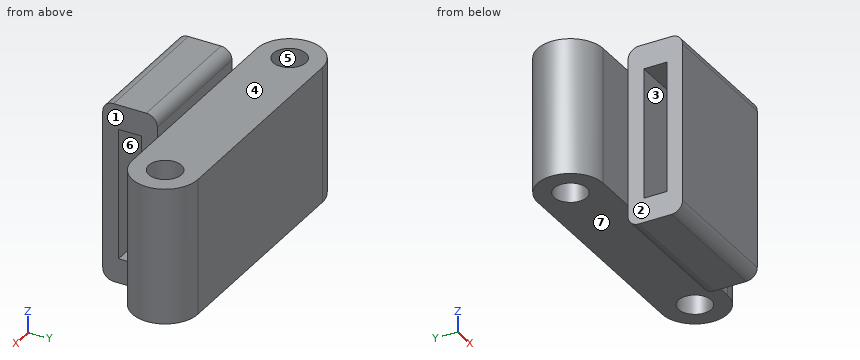
```python
from build123d import *

# Parameters (mm, degrees)
F0_W     = 12
F0_H     = 16.5
F1_DEPTH = 5
F2_R     = 1.5
F3_DEPTH = 6.25
F4_W     = 2.1
F4_H     = 12
F5_DEPTH = 12
F6_R     = 1


with BuildPart() as f1:
    # F0 (on Front) → F1 (new body)
    with BuildSketch(Plane.XZ):
        Rectangle(F0_W, F0_H)
    extrude(amount=F1_DEPTH)

    # F2 (on Top) → F3 (join, symmetric)
    with BuildSketch(Plane.XY):
        with BuildLine():
            Line((-10, 0), (10, 0))
            ThreePointArc((10, 0), (13, 3), (10, 6))
            Line((10, 6), (-10, 6))
            ThreePointArc((-10, 6), (-13, 3), (-10, 0))
        make_face()
        with Locations((-10, 3)):
            Circle(F2_R, mode=Mode.SUBTRACT)
        with Locations((10, 3)):
            Circle(F2_R, mode=Mode.SUBTRACT)
    extrude(amount=F3_DEPTH, both=True)

    # F4 (on face) → F5 (cut, through all)
    with BuildSketch(Plane(origin=(-6, 0, 0), x_dir=(0, -1, 0), z_dir=(-1, 0, 0))):
        with Locations((2.5, 0)):
            Rectangle(F4_W, F4_H)
    extrude(amount=-F5_DEPTH, mode=Mode.SUBTRACT)

    # F6
    f6_edges = [f1.edges().sort_by_distance(p)[0] for p in [
        (0, -5, 8.25),
        (0, 0, 8.25),
        (0, 0, -8.25),
        (0, -5, -8.25),
    ]]
    fillet(f6_edges, radius=F6_R)


solid = f1.part
```
Build history of the part. All positions in model axes, mm. Face numbers are marked on the shaded views. A direction names the side the tool comes from. Round coordinates to 2 decimals unless told otherwise and drop trailing zeros. Loops run counter-clockwise (first coordinate to the right, second up) from the corner with the lowest first, then second, coordinate; pieces in that order, holes last.
Item 1: Saw through at D-D (y = 3). List the corners of the cut face in (x, z), then the cut area to 3 significant figures.
Item 2: Which spindle directions (+Z, -Z, +X, -X, +Y, -Y) get a long thin tool onto all of the face, cutting with end or side? Do the marked faces 1, 2, 3 and 4. Say none if no direction does.
Item 3: Saw through at C-C (x = 5.5). List the corners of the cut face in (y, z).
Item 4: Saw through at B-B (z = 4.25). List the corners of the cut face in (x, y), then the cut area to 3 significant figures.
Item 5: Saw through at A-A (y = -3.25). List the corners of the cut face in (x, z), then the cut area to 3 significant figures.
Item 6: Pin check, flat tips, straight feed: P1, Ø6.5, axis at x = -5.5, y = 4, coming from the -Z side; P2, Ø1.2, axis at x = -9, z = 2.5, coming from the -Y side; P3, Ø5.5, axis at y = -3.5, z = -4, coming from the -X side; P4, Ø2.5, axis at x = -10, y = 3, coming from the +Z side. Stop position of each tip, or through.
Item 7: Drill centre lines: line 1 along Z through (x, y) = (-3.5, -3.5); line 2 along Y through (x, z) = (-10, -3); line 3 along X through (y, z) = (-0.75, -5.5). Where is each one in solid material? Low to high.
Item 8: Two-plate mould, pull along Z, no slides. Class the marked faces 5, 6 and 7: released by +Z, released by -Z, zero draft, split by the parting line, or undercut.
Worked answers:
1. outline: (-13, -6.25) - (-11.5, -6.25) - (-11.5, 6.25) - (-13, 6.25) - close; (-8.5, -6.25) - (8.5, -6.25) - (8.5, 6.25) - (-8.5, 6.25) - close; (11.5, -6.25) - (13, -6.25) - (13, 6.25) - (11.5, 6.25) - close
1. area: 250 mm2
2. face 1: +Z, -Z, +X, -Y
2. face 2: +Z, -Z, -X, -Y
2. face 3: +X, -X
2. face 4: +Z, +X, -X, +Y
3. outline: (-5, -7.25) arc R1 ccw to (-4, -8.25) - (-1, -8.25) arc R1 ccw to (0, -7.25) - (0, -6.25) - (6, -6.25) - (6, 6.25) - (0, 6.25) - (0, 7.25) arc R1 ccw to (-1, 8.25) - (-4, 8.25) arc R1 ccw to (-5, 7.25) - close; hole (-3.55, -6) - (-1.45, -6) - (-1.45, 6) - (-3.55, 6) - close
4. outline: (-10, 0) - (-6, 0) - (-6, -1.45) - (6, -1.45) - (6, 0) - (10, 0) arc R3 ccw to (10, 6) - (-10, 6) arc R3 ccw to start; (-6, -5) - (6, -5) - (6, -3.55) - (-6, -3.55) - close; hole circle Ø3 at (-10, 3); hole circle Ø3 at (10, 3)
4. area: 169 mm2
5. outline: (-6, -8.25) - (6, -8.25) - (6, -6) - (-6, -6) - close; (-6, 6) - (6, 6) - (6, 8.25) - (-6, 8.25) - close
5. area: 54.0 mm2
6. P1: stops at z = -6.25
6. P2: stops at y = 0
6. P3: stops at x = -6
6. P4: passes through
7. line 1: z = -8.25 to -6, 6 to 8.25
7. line 2: y = 0 to 1.5, 4.5 to 6
7. line 3: x = -6 to 6
8. face 5: zero draft
8. face 6: undercut
8. face 7: released by -Z
